from build123d import *

# Parameters (mm, degrees)
SKETCH_1_R           = 21
EXTRUDE_1_DEPTH      = 110
SKETCH_2_W           = 8
SKETCH_2_H           = 8
EXTRUDE_2_DEPTH      = 0.1
EXTRUDE_2_DEPTH_BACK = 55
SKETCH_3_R           = 175
EXTRUDE_3_DEPTH      = 15
SKETCH_4_R           = 125
SKETCH_4_R_2         = 116
EXTRUDE_4_DEPTH      = 5
SKETCH_5_R           = 116
SKETCH_5_R_2         = 40
CUT_EXTRUDE_1_DEPTH  = 8
CHAMFER_1_SIZE       = 1
SKETCH_6_R           = 9.5
CUT_EXTRUDE_2_DEPTH  = 16
SKETCH_7_R           = 125
EXTRUDE_5_DEPTH      = 68
SKETCH_8_R           = 140
EXTRUDE_6_DEPTH      = 292
SKETCH_9_R           = 144
EXTRUDE_7_DEPTH      = 145
CHAMFER_2_SIZE       = 60
EXTRUDE_8_DEPTH      = 228
CUT_EXTRUDE_3_REACH  = 337
SKETCH_11_R          = 7.5
SKETCH_12_W          = 120
SKETCH_12_H          = 120
EXTRUDE_9_DEPTH      = 245
SKETCH_13_R          = 35
EXTRUDE_10_DEPTH     = 150
CHAMFER_3_SIZE       = 1
SKETCH_15_R          = 12
SKETCH_16_R          = 16
EXTRUDE_11_DEPTH     = 14
EXTRUDE_12_DEPTH     = 16
SKETCH_18_R          = 7
CUT_EXTRUDE_4_DEPTH  = 16


with BuildPart() as part:
    # Эскиз1 → Вытянуть1 (new body)
    with BuildSketch(Plane.XY):
        Circle(SKETCH_1_R)
    extrude(amount=EXTRUDE_1_DEPTH)

    # Эскиз2 → Вытянуть2 (add, two sides)
    with BuildSketch(Plane(origin=(0, 0, 0), x_dir=(-1, 0, 0), z_dir=(0, 0, -1))) as extrude_2_sk:
        with Locations((0, 20)):
            Rectangle(SKETCH_2_W, SKETCH_2_H)
    extrude(amount=EXTRUDE_2_DEPTH)
    extrude(extrude_2_sk.sketch, amount=-EXTRUDE_2_DEPTH_BACK)

    # Эскиз3 → Вытянуть3 (add)
    with BuildSketch(Plane.XY.offset(110)):
        Circle(SKETCH_3_R)
    extrude(amount=EXTRUDE_3_DEPTH)

    # Эскиз4 → Вытянуть4 (add)
    with BuildSketch(Plane(origin=(0, 0, 110), x_dir=(-1, 0, 0), z_dir=(0, 0, -1))):
        with Locations(Location((0, 0, 0), (0, 0, 180))):  # turned: the seam where the file's is
            Circle(SKETCH_4_R)
        Circle(SKETCH_4_R_2, mode=Mode.SUBTRACT)
    extrude(amount=EXTRUDE_4_DEPTH)

    # Эскиз5 → Вырез-Вытянуть1 (cut)
    with BuildSketch(Plane(origin=(0, 0, 110), x_dir=(-1, 0, 0), z_dir=(0, 0, -1))):
        Circle(SKETCH_5_R)
        Circle(SKETCH_5_R_2, mode=Mode.SUBTRACT)
    extrude(amount=-CUT_EXTRUDE_1_DEPTH, mode=Mode.SUBTRACT)

    # Фаска1
    chamfer_1_edges = [part.edges().sort_by_distance(p)[0] for p in [
        (-125, 0, 105),
        (40, 0, 110),
        (-13.360389216, -16.201851746, 0),
    ]]
    chamfer(chamfer_1_edges, length=CHAMFER_1_SIZE)

    # Эскиз6 → Вырез-Вытянуть2 (cut, through all)
    with BuildSketch(Plane(origin=(0, 0, 110), x_dir=(-1, 0, 0), z_dir=(0, 0, -1))):
        with Locations((-57.402514855, 138.581929877)):
            Circle(SKETCH_6_R)
        with Locations((57.402514855, 138.581929877)):
            Circle(SKETCH_6_R)
        with Locations((138.581929877, 57.402514855)):
            Circle(SKETCH_6_R)
        with Locations((138.581929877, -57.402514855)):
            Circle(SKETCH_6_R)
        with Locations((57.402514855, -138.581929877)):
            Circle(SKETCH_6_R)
        with Locations((-57.402514855, -138.581929877)):
            Circle(SKETCH_6_R)
        with Locations((-138.581929877, -57.402514855)):
            Circle(SKETCH_6_R)
        with Locations((-138.581929877, 57.402514855)):
            Circle(SKETCH_6_R)
    extrude(amount=-CUT_EXTRUDE_2_DEPTH, mode=Mode.SUBTRACT)

    # Эскиз7 → Вытянуть5 (add)
    with BuildSketch(Plane.XY.offset(125)):
        Circle(SKETCH_7_R)
    extrude(amount=EXTRUDE_5_DEPTH)

    # Эскиз8 → Вытянуть6 (add)
    with BuildSketch(Plane.XY.offset(193)):
        Circle(SKETCH_8_R)
    extrude(amount=EXTRUDE_6_DEPTH)

    # Эскиз9 → Вытянуть7 (add)
    with BuildSketch(Plane.XY.offset(485)):
        Circle(SKETCH_9_R)
    extrude(amount=EXTRUDE_7_DEPTH)

    # Фаска2
    chamfer_2_edges = [part.edges().sort_by_distance(p)[0] for p in [
        (-144, 0, 630),
    ]]
    chamfer(chamfer_2_edges, length=CHAMFER_2_SIZE)

    # Эскиз10 → Вытянуть8 (add)
    with BuildSketch(Plane(origin=(0, 0, 193), x_dir=(-1, 0, 0), z_dir=(0, 0, -1))):
        Polygon((-152, -160), (-91.607695155, -160), (-51.945448858, -91.302974272), (-67.533906126, -82.302974272), (-102, -142), (-152, -142), align=None)
        Polygon((91.607695155, -160), (51.945448858, -91.302974272), (67.533906126, -82.302974272), (102, -142), (152, -142), (152, -160), align=None)
    extrude(amount=-EXTRUDE_8_DEPTH)

    # Эскиз11 → Вырез-Вытянуть3 (cut, up to next)
    with BuildSketch(Plane.XZ.offset(160), mode=Mode.PRIVATE) as cut_extrude_3_sk1:
        with Locations((-127, 218)):
            Circle(SKETCH_11_R)
    cut_extrude_3_tool1 = extrude(cut_extrude_3_sk1.sketch, amount=-CUT_EXTRUDE_3_REACH, mode=Mode.PRIVATE) & part.part
    add(cut_extrude_3_tool1.solids().sort_by_distance((-127, -160, 218))[0], mode=Mode.SUBTRACT)
    # Эскиз11 → Вырез-Вытянуть3 (cut, up to next)
    with BuildSketch(Plane.XZ.offset(160), mode=Mode.PRIVATE) as cut_extrude_3_sk2:
        with Locations((127, 218)):
            Circle(SKETCH_11_R)
    cut_extrude_3_tool2 = extrude(cut_extrude_3_sk2.sketch, amount=-CUT_EXTRUDE_3_REACH, mode=Mode.PRIVATE) & part.part
    add(cut_extrude_3_tool2.solids().sort_by_distance((127, -160, 218))[0], mode=Mode.SUBTRACT)
    # Эскиз11 → Вырез-Вытянуть3 (cut, up to next)
    with BuildSketch(Plane.XZ.offset(160), mode=Mode.PRIVATE) as cut_extrude_3_sk3:
        with Locations((-127, 396)):
            Circle(SKETCH_11_R)
    cut_extrude_3_tool3 = extrude(cut_extrude_3_sk3.sketch, amount=-CUT_EXTRUDE_3_REACH, mode=Mode.PRIVATE) & part.part
    add(cut_extrude_3_tool3.solids().sort_by_distance((-127, -160, 396))[0], mode=Mode.SUBTRACT)
    # Эскиз11 → Вырез-Вытянуть3 (cut, up to next)
    with BuildSketch(Plane.XZ.offset(160), mode=Mode.PRIVATE) as cut_extrude_3_sk4:
        with Locations((127, 396)):
            Circle(SKETCH_11_R)
    cut_extrude_3_tool4 = extrude(cut_extrude_3_sk4.sketch, amount=-CUT_EXTRUDE_3_REACH, mode=Mode.PRIVATE) & part.part
    add(cut_extrude_3_tool4.solids().sort_by_distance((127, -160, 396))[0], mode=Mode.SUBTRACT)

    # Эскиз12 → Вытянуть9 (add)
    with BuildSketch(Plane(origin=(0, 0, 0), x_dir=(1, 0, 0), z_dir=(0, 1, 0))):
        with Locations((0, -254)):
            Rectangle(SKETCH_12_W, SKETCH_12_H)
    extrude(amount=EXTRUDE_9_DEPTH)

    # Эскиз13 → Вытянуть10 (add)
    with BuildSketch(Plane(origin=(0, 0, 0), x_dir=(1, 0, 0), z_dir=(0, 1, 0))):
        with Locations(Location((0, -371, 0), (0, 0, 90))):  # turned: the seam where the file's is
            Circle(SKETCH_13_R)
    extrude(amount=EXTRUDE_10_DEPTH)

    # Фаска3
    chamfer_3_edges = [part.edges().sort_by_distance(p)[0] for p in [
        (0, 150, 406),
    ]]
    chamfer(chamfer_3_edges, length=CHAMFER_3_SIZE)

    # По траектории1: sweep along a path in Эскиз14
    with BuildLine(Plane.XY.offset(370)) as sweep_1_path:
        CenterArc((0, 188), 38, 0, 360)
    # Эскиз15 → По траектории1 (sweep)
    with BuildSketch(Plane(origin=(0, 0, 0), x_dir=(0, 0, -1), z_dir=(1, 0, 0))):
        with Locations((-370, 226)):
            Circle(SKETCH_15_R)
    sweep(path=sweep_1_path.line)

    # Эскиз16 → Вытянуть11 (add)
    with BuildSketch(Plane.ZY.offset(60)):
        with Locations(Location((254, 185, 0), (0, 0, 180))):  # turned: the seam where the file's is
            Circle(SKETCH_16_R)
    extrude(amount=EXTRUDE_11_DEPTH)

    # Эскиз17 → Вытянуть12 (add)
    with BuildSketch(Plane.ZY.offset(74)):
        Polygon((254, 207.516660498), (234.5, 196.258330249), (234.5, 173.741669751), (254, 162.483339502), (273.5, 173.741669751), (273.5, 196.258330249), align=None)
    extrude(amount=EXTRUDE_12_DEPTH)

    # Эскиз18 → Вырез-Вытянуть4 (cut)
    with BuildSketch(Plane.ZY.offset(90)):
        with Locations((254, 185)):
            Circle(SKETCH_18_R)
    extrude(amount=-CUT_EXTRUDE_4_DEPTH, mode=Mode.SUBTRACT)


solid = part.part
Geometry check sheet. Reference: the model listing, model coordinates, mm. A direction names the side the tool comes from. Give positions to 0.01 mm unless a question says otherwise; leave off trailing zeros. Order: outer loops, then holes, each group sorted by start corner. A loop starts at its lowest first (then second) coordinate and runs counter-clockwise, first axis right, second up. Notation, with made-up numbers: (-6.5, 51) - (16.5, 51) arc R30 cw to (16.5, 84) - close; hole circle Ø7 at (-21.5, 69). An arc over 180 degrees is marked (long way). Answer as a JSON object with one key per item and string values.
(1) Cross-section at A-A (z = 218). Record the cut outline in (x, y), then the cut area to 3 significant figures.
Report:
{"outline": "(-152, -160) - (-134.5, -160) - (-134.5, -142) - (-152, -142) - close; (-119.5, -160) - (-91.61, -160) - (-69.42, -121.57) arc R140 ccw to (69.42, -121.57) - (91.61, -160) - (119.5, -160) - (119.5, -142) - (102, -142) - (84.47, -111.64) arc R140 ccw to (60, 126.49) - (60, 245) - (-60, 245) - (-60, 126.49) arc R140 ccw to (-84.47, -111.64) - (-102, -142) - (-119.5, -142) - close; (134.5, -160) - (152, -160) - (152, -142) - (134.5, -142) - close", "area": "77,600 mm^2"}
(2) Cross-section at B-B (z = 371). Record the cut outline in (x, y).
Report:
{"outline": "(-152, -160) - (-91.61, -160) - (-69.42, -121.57) arc R140 ccw to (69.42, -121.57) - (91.61, -160) - (152, -160) - (152, -142) - (102, -142) - (84.47, -111.64) arc R140 ccw to (35, 135.55) - (35, 149) - (34, 150) - (32.43, 150) arc R49.96 ccw (long way) to (-32.43, 150) - (-34, 150) - (-35, 149) - (-35, 135.55) arc R140 ccw to (-84.47, -111.64) - (-102, -142) - (-152, -142) - close; hole circle Ø52.08 at (0, 188)"}
(3) Tool access check on faces 1 (the flat face through (-1, 245, 253)), 2 (the flat face through (-90, 185, 245)), 3 (the flat face through (-74, 170, 248)), 4 (the flat face through (-82, 185, 273.5)), 5 (the flat face through (-81.89, 201.97, 244.39)). Record the directions out of +Z, -Z, +X, -X, +Y, -Y that give a thin tool (end or side, any length) a straight path to the whole face; none if there is none.
Report:
{"face 1": "+Z, -Z, +X, -X, +Y", "face 2": "+Z, -Z, -X, +Y", "face 3": "none", "face 4": "+Z, -X, +Y", "face 5": "-Z, -X, +Y"}
(4) Depth check by flat-ended pin: pin 1 Ø11.5 at (x, y) = (57.4, -138.58) entering from -Z; pin 2 Ø2 at (x, z) = (101, 188) entering from +Y; pin 3 Ø18 at (x, z) = (116.5, 350) entering from -Y; pin 4 Ø2.5 at (y, z) = (18.5, 25) entering from -X. Enter the tip coordinate at first touch or a pass-through.
Report:
{"pin 1": "through", "pin 2": "y = 75", "pin 3": "y = -160", "pin 4": "x = -11.98"}
(5) Draft check along X on faces 6 (the flat face through (122, -160, 305)), 7 (the flat face through (152, -151, 305)), 8 (the cylindrical face through (59.462, -147.856, 117.395)). Enter one of: released by +X, released by -X, zero draft, split by the parting line, or undercut.
Report:
{"face 6": "zero draft", "face 7": "released by +X", "face 8": "undercut"}
(6) Material ranges on line 1 (Z direction, x = -127, y = -147.5); line 2 (X direction, y = 171.5, z = 206); line 3 (Z direction, x = -113, y = 102.5), recorded low to high.
Report:
{"line 1": "193 to 210.5, 225.5 to 388.5, 403.5 to 421", "line 2": "-60 to 60", "line 3": "110 to 125"}
(7) Cross-section at C-C (z = 588). Record the cut outline in (x, y).
Report:
{"outline": "circle Ø252 at (0, 0)"}
